Source: CAD feature listing. Evaluate the final solid. Frame: model axes, mm. A direction names the side the tool comes from. Give positions to 0.01 mm unless a question says otherwise; leave off trailing zeros. Write each loop counter-clockwise with the first axis right and the second up, starting at its lowest first coordinate (ties: lowest second). Pieces come first, ordered by that corner, then holes. Notation, with made-up numbers: (-22.5, -27) -> (-1.5, -27) arc R17 cw to (-1.5, -5) -> close; hole circle Ø2 at (33, 39.5). An arc over 180 degrees is marked (long way). Use one line per item in the form item = value. Start each with the question number.
(1) Cut plane A-A, the plane z = 11. Output: boundary loops of the cut face in (x, y), and give its area (3 significant figures).
(2) Cut plane B-B, the plane y = 0. Output: boundary loops of the cut face in (x, z).
(3) First-contact query: P1, Ø3.5, axis at x = -1, z = 11, coming from the -Y side; P2, Ø9, axis at x = 0, y = 0, coming from the -Z side; P3, Ø1.6, axis at y = 32, z = 13, coming from the +X side; P4, Ø4, axis at x = 19.5, z = 7, coming from the -Y side. Flat tips, straight axial feed; report the tip coordinate or a pass-through.
(4) Cut plane D-D, the plane z = 7. Output: boundary loops of the cut face in (x, y).
(5) Set-up query: faces 4 (the face through (-4.249, -19.134, 10.994)), 5 (the face through (29.766, 25.523, 11.238)), 6 (the face through (13, 37, 11.94)). Return all of +Z, -Z, +X, -X, +Y, -Y with unobstructed straight access to the full face (end or side cutting, diameter ignored); none if empty.
(6) Draft query along Y for faces 1 (the face through (19.17, -6.04, 12.96)), 2 (the face through (31.085, 22.6, 11.731)), 3 (the face through (0, 0, 0)). Return one class per face: pulls with the +Y half, pulls with the -Y half, needs draft (parallel to the pull), parting line crosses it, or undercut.
(7) Material intervals for line 1 along X through (y, z) = (0, 8.25); line 2 along Y through (x, z) = (0, 11.2); line 3 along Y through (x, z) = (0, 13), sorted ascending. Write a range as from..to.
Solid Edge part; units mm, degrees
sketch "Sketch1" plane through (0, 0, 0) normal (0, 0, 1) x (1, 0, 0)
  line L0 (27.5, 27.5) -> (-27.5, 27.5)
  line L1 (-27.5, 27.5) -> (-27.5, -27.5)
  line L2 (-27.5, -27.5) -> (27.5, -27.5)
  line L3 (27.5, -27.5) -> (27.5, 27.5)
extrude "Protrusion1" add sketch "Sketch1" along normal blind 13.94
sketch "Sketch2" plane through (0, 0, 0) normal (0, -1, 0) x (1, 0, 0)
  line L0 (20.1, 13.94) -> (20.1, 12)
  line L1 (19.6, 12) -> (20.1, 12)
  line L2 (19.6, 9.96) -> (19.6, 12)
  line L3 (7.6, 9.96) -> (19.6, 9.96)
  line L4 (7.6, 9.96) -> (7.6, 1.46)
  line L5 (7.6, 1.46) -> (0, 1.46)
  line L6 (0, 13.94) -> (0, 1.46)
  line L7 (20.1, 13.94) -> (0, 13.94)
revolve "RevolvedCutout1" cut sketch "Sketch2" angle 360 about axis through (0, 0, 13.94) along (0, 0, -1)
sketch "Sketch3" plane through (0, 0, 6.97) normal (0, -1, 0) x (1, 0, 0)
  line L0 (9.1, 1.49) -> (39.1, 1.49)
  line L1 (39.1, 1.49) -> (39.1, -6.97)
  line L2 (39.1, -6.97) -> (9.1, -6.97)
  line L3 (9.1, -6.97) -> (9.1, 1.49)
revolve "RevolvedCutout2" cut sketch "Sketch3" angle 360 about axis through (0, 0, 12.8514) along (0, 0, -1)
sketch "Sketch4" plane through (0, 0, 13.94) normal (0, 0, 1) x (-1, 0, 0)
  line L0 (-35.2782, -26.7929) -> (-26.7929, -35.2782)
  line L1 (-26.7929, -35.2782) -> (-19.0147, -27.5)
  line L2 (-19.0147, -27.5) -> (-21.136, -27.5)
  line L3 (-26.7929, -33.1569) -> (-21.136, -27.5)
  line L4 (-27.8536, -32.0962) -> (-26.7929, -33.1569)
  line L5 (-23.2574, -27.5) -> (-27.8536, -32.0962)
  line L6 (-27.5, -27.5) -> (-23.2574, -27.5)
  line L7 (-27.5, -23.2574) -> (-27.5, -27.5)
  line L8 (-27.5, -23.2574) -> (-32.0962, -27.8536)
  line L9 (-33.1569, -26.7929) -> (-32.0962, -27.8536)
  line L10 (-27.5, -21.136) -> (-33.1569, -26.7929)
  line L11 (-27.5, -19.0147) -> (-27.5, -21.136)
  line L12 (-35.2782, -26.7929) -> (-27.5, -19.0147)
extrude "Protrusion2" add sketch "Sketch4" against normal up to vertex (5.48 mm away)
sketch "Sketch5" plane through (3.8891, 3.8891, 13.94) normal (0, 0, 1) x (0, 1, 0)
  line L0 (32.1109, 22.8891) -> (25.1109, 22.8891)
  line L1 (25.1109, 22.8891) -> (25.1109, 29.8891)
  line L2 (25.1109, 29.8891) -> (32.1109, 29.8891)
  line L3 (32.1109, 29.8891) -> (32.1109, 22.8891)
  line L4 (33.6109, 21.3891) -> (23.6109, 21.3891)
  line L5 (23.6109, 21.3891) -> (23.6109, 31.3891)
  line L6 (23.6109, 31.3891) -> (33.6109, 31.3891)
  line L7 (33.6109, 31.3891) -> (33.6109, 21.3891)
  line L8 (32.1109, -6.6256) -> (25.1109, -6.6256)
  line L9 (25.1109, -6.6256) -> (25.1109, -13.6256)
  line L10 (25.1109, -13.6256) -> (32.1109, -13.6256)
  line L11 (32.1109, -13.6256) -> (32.1109, -6.6256)
  line L12 (33.6109, -5.1256) -> (23.6109, -5.1256)
  line L13 (23.6109, -5.1256) -> (23.6109, -15.1256)
  line L14 (23.6109, -15.1256) -> (33.6109, -15.1256)
  line L15 (33.6109, -15.1256) -> (33.6109, -5.1256)
  line L16 (-32.8891, -15.1109) -> (-39.8891, -15.1109)
  line L17 (-39.8891, -15.1109) -> (-39.8891, -22.1109)
  line L18 (-39.8891, -22.1109) -> (-32.8891, -22.1109)
  line L19 (-32.8891, -22.1109) -> (-32.8891, -15.1109)
  line L20 (-31.3891, -13.6109) -> (-41.3891, -13.6109)
  line L21 (-41.3891, -13.6109) -> (-41.3891, -23.6109)
  line L22 (-41.3891, -23.6109) -> (-31.3891, -23.6109)
  line L23 (-31.3891, -23.6109) -> (-31.3891, -13.6109)
  line L24 (-39.8891, 22.8891) -> (-32.8891, 22.8891)
  line L25 (-32.8891, 22.8891) -> (-32.8891, 29.8891)
  line L26 (-32.8891, 29.8891) -> (-39.8891, 29.8891)
  line L27 (-39.8891, 29.8891) -> (-39.8891, 22.8891)
  line L28 (-41.3891, 21.3891) -> (-31.3891, 21.3891)
  line L29 (-31.3891, 21.3891) -> (-31.3891, 31.3891)
  line L30 (-31.3891, 31.3891) -> (-41.3891, 31.3891)
  line L31 (-41.3891, 31.3891) -> (-41.3891, 21.3891)
extrude "Protrusion3" add sketch "Sketch5" against normal blind 2
fillet "Round_1" radius 5 3 edges at (-27.5, 27.5, 10.2) (-27.5, -27.5, 10.2) (27.5, -27.5, 10.2)
fillet "Round_2" radius 1 28 edges at (-27.5, 37.5, 12.94) (-17.5, 37.5, 12.94) (-26, 36, 12.94) (-19, 36, 12.94) (-26, 29, 12.94) (-19, 29, 12.94) (-17.5, 27.5, 12.94) (10.5147, 29, 12.94) (17.5147, 29, 12.94) (10.5147, 36, 12.94) (17.5147, 36, 12.94) (9.0147, 37.5, 12.94) (19.0147, 37.5, 12.94) (9.0147, 27.5, 12.94) (-26, -29, 12.94) (-26, -36, 12.94) (-19, -36, 12.94) (-19, -29, 12.94) (-17.5, -27.5, 12.94) (-17.5, -37.5, 12.94) (-27.5, -37.5, 12.94) (19, -29, 12.94) (19, -36, 12.94) (26, -36, 12.94) (26, -29, 12.94) (27.5, -37.5, 12.94) (17.5, -37.5, 12.94) (17.5, -27.5, 12.94)
fillet "Round_3" radius 1 13 edges at (-9.1, 0, 0) (0, -27.5, 8.46) (26.0355, -26.0355, 8.46) (27.5, -1.7426, 8.46) (-26.0355, -26.0355, 8.46) (-27.5, 0, 8.46) (-26.0355, 26.0355, 8.46) (-1.7426, 27.5, 8.46) (31.3891, 22.9038, 8.46) (31.0355, 31.0355, 8.46) (22.9038, 31.3891, 8.46) (35.2782, 26.7929, 11.2) (26.7929, 35.2782, 11.2)
Geometry says:
q1.outline = (-27.5, -22.5) arc R5 ccw to (-22.5, -27.5) -> (22.5, -27.5) arc R5 ccw to (27.5, -22.5) -> (27.5, 19.01) -> (34.57, 26.09) arc R1 ccw to (34.57, 27.5) -> (27.5, 34.57) arc R1 ccw to (26.09, 34.57) -> (19.01, 27.5) -> (-22.5, 27.5) arc R5 ccw to (-27.5, 22.5) -> close; hole circle Ø39.2 at (0, 0); hole (21.14, 27.5) -> (23.26, 27.5) -> (27.85, 32.1) -> (26.79, 33.16) -> close; hole (27.5, 21.14) -> (33.16, 26.79) -> (32.1, 27.85) -> (27.5, 23.26) -> close
q1.area = 1,880 mm^2
q2.outline = (-27.5, 9.46) arc R1 ccw to (-26.5, 8.46) -> (-9.1, 8.46) -> (-9.1, 1) arc R1 ccw to (-8.1, 0) -> (8.1, 0) arc R1 ccw to (9.1, 1) -> (9.1, 8.46) -> (26.5, 8.46) arc R1 ccw to (27.5, 9.46) -> (27.5, 13.94) -> (20.1, 13.94) -> (20.1, 12) -> (19.6, 12) -> (19.6, 9.96) -> (7.6, 9.96) -> (7.6, 1.46) -> (-7.6, 1.46) -> (-7.6, 9.96) -> (-19.6, 9.96) -> (-19.6, 12) -> (-20.1, 12) -> (-20.1, 13.94) -> (-27.5, 13.94) -> close
q3.P1 = -27.5
q3.P2 = 0
q3.P3 = 30.87
q3.P4 = -27.39
q4.outline = circle Ø18.2 at (0, 0); hole circle Ø15.2 at (0, 0)
q5.face_4 = +Z
q5.face_5 = +Z, -Z
q5.face_6 = -Z, -X, +Y
q6.face_1 = undercut
q6.face_2 = pulls with the -Y half
q6.face_3 = needs draft
q7.line_1 = -9.1..-7.6, 7.6..9.1
q7.line_2 = -27.5..-19.6, 19.6..27.5
q7.line_3 = -27.5..-20.1, 20.1..27.5
